Source: CAD feature listing. Evaluate the final solid. Frame: model axes, mm. Face numbers are marked on the shaded views. A direction names the side the tool comes from. Give positions to 0.01 mm unless a question says otherwise; leave off trailing zeros. Loops run counter-clockwise (first coordinate to the right, second up) from the corner with the lowest first, then second, coordinate; pieces in that order, holes last. Notation, with made-up numbers: M 70.5,-28 L 123.5,-28 A12 ccw 123.5,-5 Z; hole C 28,-1.5 d6. An arc over 180 degrees is marked long. Put each result on its own line as item: value.
from build123d import *

# Parameters (mm, degrees)
F0_W      = 63.5
F0_H      = 15.24
F0_R      = 3.937
F0_H_2    = 38.1
F0_R_2    = 7.4295
F0_H_3    = 35.56
F1_DEPTH  = 19.05
F5_DEPTH  = 50.8
F7_DEPTH  = 3.175
F2_R      = 11.3792
F9_DEPTH  = 3.175
F6_R      = 7.4295
F10_DEPTH = 19.05
F11_DEPTH = 73.661
F8_R      = 5.08
F12_DEPTH = 31.75


# Not quite as in the source:
# - a feature names something its author has since deleted; it is built from what else it names


with BuildPart() as f1:
    # F0 (on Top) → F1 (new body)
    with BuildSketch(Plane.XY):
        with Locations((31.75, 81.28)):
            Rectangle(F0_W, F0_H)
        with Locations((11.43, 81.28)):
            Circle(F0_R, mode=Mode.SUBTRACT)
        with Locations((52.07, 81.28)):
            Circle(F0_R, mode=Mode.SUBTRACT)
        with Locations((31.75, 54.61)):
            Rectangle(F0_W, F0_H_2)
        with Locations((13.5382, 59.944)):
            Circle(F0_R_2, mode=Mode.SUBTRACT)
        with Locations((49.9618, 59.944)):
            Circle(F0_R_2, mode=Mode.SUBTRACT)
        with Locations((13.5382, 59.944)):
            Circle(F0_R_2)
        with Locations((49.9618, 59.944)):
            Circle(F0_R_2)
        with Locations((31.75, 17.78)):
            Rectangle(F0_W, F0_H_3)
        with Locations((31.75, 11.176)):
            Circle(F0_R, mode=Mode.SUBTRACT)
    extrude(amount=F1_DEPTH)


with BuildPart() as f3_1:
    # F3: copy of F1
    add(f1.part.moved(Location((-152.4, 0, 0))))


with BuildPart() as f1_1:
    add(f1.part)

    # F0 (on Top) → F5 (join)
    with BuildSketch(Plane.XY):
        with Locations((31.75, 54.61)):
            Rectangle(F0_W, F0_H_2)
        with Locations((13.5382, 59.944)):
            Circle(F0_R_2, mode=Mode.SUBTRACT)
        with Locations((49.9618, 59.944)):
            Circle(F0_R_2, mode=Mode.SUBTRACT)
        with Locations((49.9618, 59.944)):
            Circle(F0_R_2)
        with Locations((13.5382, 59.944)):
            Circle(F0_R_2)
    extrude(amount=F5_DEPTH)

    # F0 (on Top) → F7 (cut)
    with BuildSketch(Plane.XY):
        with Locations((49.9618, 59.944)):
            Circle(F0_R_2)
        with Locations((13.5382, 59.944)):
            Circle(F0_R_2)
    extrude(amount=F7_DEPTH, mode=Mode.SUBTRACT)

    # F2 (on face) → F9 (cut)
    with BuildSketch(Plane(origin=(0, 0, 0), x_dir=(1, 0, 0), z_dir=(0, 0, -1))):
        with Locations((49.9618, -59.944)):
            Circle(F2_R)
        with Locations((13.5382, -59.944)):
            Circle(F2_R)
    extrude(amount=-F9_DEPTH, mode=Mode.SUBTRACT)

    # F6 (on face) → F10 (cut)
    with BuildSketch(Plane(origin=(0, 73.66, 0), x_dir=(-1, 0, 0), z_dir=(0, 1, 0))):
        with Locations((-49.9618, 38.1)):
            Circle(F6_R)
    extrude(amount=-F10_DEPTH, mode=Mode.SUBTRACT)

    # F6 (on face) → F11 (cut, through all)
    with BuildSketch(Plane(origin=(0, 73.66, 0), x_dir=(-1, 0, 0), z_dir=(0, 1, 0))):
        with Locations((-13.5382, 38.1)):
            Circle(F6_R)
    extrude(amount=-F11_DEPTH, mode=Mode.SUBTRACT)

    # F8 (on face) → F12 (cut)
    with BuildSketch(Plane(origin=(0, 0, 3.175), x_dir=(1, 0, 0), z_dir=(0, 0, -1))):
        with Locations((49.9618, -59.944)):
            Circle(F8_R)
    extrude(amount=-F12_DEPTH, mode=Mode.SUBTRACT)


solid = f1_1.part
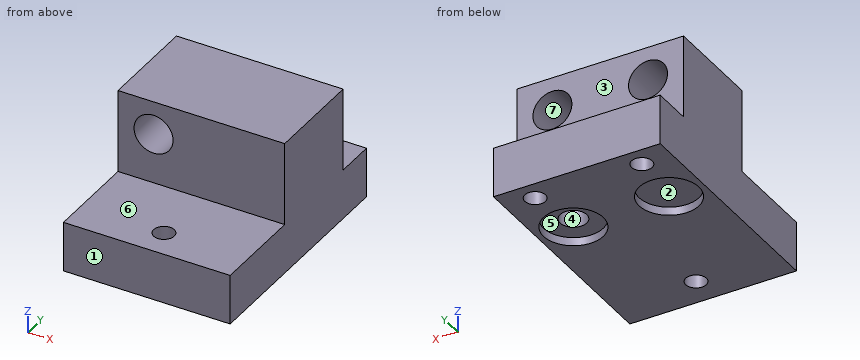
1. Material intervals for line 1 (Y direction, x = 40, z = 47.5); line 2 (X direction, y = 64, z = 10); line 3 (X direction, y = 58, z = 27.5), sorted ascending. Write a range as from..to.
Found:
line 1: 35.56..73.66
line 2: 0..46.9, 53.02..63.5
line 3: 0..45.27, 54.66..63.5
2. Draft query along Y for the marked faces 1, 2, 3 and 4. Return one class per face: pulls with the +Y half, pulls with the -Y half, needs draft (parallel to the pull), parting line crosses it, or undercut.
Found:
face 1: pulls with the -Y half
face 2: undercut
face 3: pulls with the +Y half
face 4: undercut
3. Section query B-B (z = 38.1). Output: boundary loops of the cut face in (x, y), plus the area to 3 significant figures.
Found:
outline: M 0,35.56 L 6.11,35.56 L 6.11,73.66 L 0,73.66 Z; M 20.97,35.56 L 63.5,35.56 L 63.5,73.66 L 57.39,73.66 L 57.39,54.61 L 42.53,54.61 L 42.53,73.66 L 20.97,73.66 Z
area: 1,570 mm^2
4. Section query D-D (x = 11.43). Output: boundary loops of the cut face in (y, z) (3 decimals), plus the area to 3 significant figures.
Found:
outline: M 0,0 L 48.762,0 L 48.762,3.175 L 71.126,3.175 L 71.126,0 L 77.343,0 L 77.343,19.05 L 73.66,19.05 L 73.66,30.976 L 35.56,30.976 L 35.56,19.05 L 0,19.05 Z; M 35.56,45.224 L 73.66,45.224 L 73.66,50.8 L 35.56,50.8 Z; M 85.217,0 L 88.9,0 L 88.9,19.05 L 85.217,19.05 Z
area: 2,140 mm^2
5. Contact query for flat-ended pins moving along their axis: P1, Ø13.5, axis at x = 13.54, y = 59.94, coming from the -Z side (3 decimals); P2, Ø12, axis at x = 10, z = 38.5, coming from the +Y side; P3, Ø18, axis at x = 35, y = 19, coming from the +Z side. Output: stop coordinate, or through.
Found:
P1: z = 3.175
P2: y = 73.66
P3: z = 19.05
6. Section query A-A (y = 81.28). Output: boundary loops of the cut face in (x, z).
Found:
outline: M 0,0 L 7.49,0 L 7.49,19.05 L 0,19.05 Z; M 15.37,0 L 48.13,0 L 48.13,19.05 L 15.37,19.05 Z; M 56.01,0 L 63.5,0 L 63.5,19.05 L 56.01,19.05 Z
7. Section query C-C (x = 31.75). Output: boundary loops of the cut face in (y, z), plus the area to 3 significant figures.
Found:
outline: M 0,0 L 7.24,0 L 7.24,19.05 L 0,19.05 Z; M 15.11,0 L 88.9,0 L 88.9,19.05 L 73.66,19.05 L 73.66,50.8 L 35.56,50.8 L 35.56,19.05 L 15.11,19.05 Z
area: 2,750 mm^2
8. Access query for the marked faces 5, 6 and 7. Directions: +Z, -Z, +X, -X, +Y, -Y. A direction counts if a zero-diameter tool reaches every point of the face in a straight line with its end or side. Return the directions, or none.
Found:
face 5: -Z
face 6: +Z, +X, -X, -Y
face 7: +Y
